Could you check a few things on this model? Use its own coordinates, in mm. Face numbers are marked on the shaded views. A direction names the side the tool comes from. Give positions to 0.01 mm unless a question says otherwise; leave off trailing zeros. Write each loop counter-clockwise with the first axis right and the second up, starting at its lowest first coordinate (ties: lowest second). Pieces come first, ordered by that corner, then holes. Notation, with made-up numbers: M -39.5,75.25 L 7.5,75.25 A11 cw 7.5,84.25 Z; hole C 25,-26.75 d1. An arc over 180 degrees is marked long. Use one line per item in the form item = value.
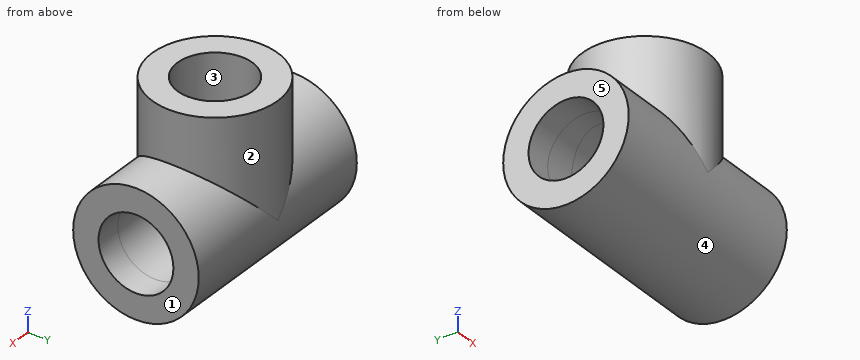
from build123d import *

# Parameters (mm, degrees)
F0_R          = 19
F0_R_2        = 11.335
F1_DEPTH      = 33
F1_DEPTH_BACK = 33
F2_R          = 19
F2_R_2        = 11.335
F3_DEPTH      = 34.5
F4_DEPTH      = 25
F4_DEPTH_BACK = 25


with BuildPart() as f1:
    # F0 (on Right) → F1 (new body, two sides)
    with BuildSketch(Plane.YZ) as f1_sk:
        Circle(F0_R)
        Circle(F0_R_2, mode=Mode.SUBTRACT)
    extrude(amount=F1_DEPTH)
    extrude(f1_sk.sketch, amount=-F1_DEPTH_BACK)

    # F2 (on Top) → F3 (join)
    with BuildSketch(Plane.XY):
        Circle(F2_R)
        Circle(F2_R_2, mode=Mode.SUBTRACT)
    extrude(amount=F3_DEPTH)

    # F0 (on Right) → F4 (cut, two sides)
    with BuildSketch(Plane.YZ) as f4_sk:
        Circle(F0_R_2)
    extrude(amount=-F4_DEPTH, mode=Mode.SUBTRACT)
    extrude(f4_sk.sketch, amount=F4_DEPTH_BACK, mode=Mode.SUBTRACT)


solid = f1.part
1) If I drill on L1, parallel to Z at x = 9.5, y = 0 (3 decimals), over which ranges is the centre line in solid material (lowest first)?
Checked values:
L1 = -19 to -11.335, 11.335 to 19
2) Thinking about a two-plate mould opening in Y: for the marked faces 1, 2 and 3, which applies, released by +Y, released by -Y, zero draft, split by the parting line, or undercut?
Checked values:
face_1 = zero draft
face_2 = split by the parting line
face_3 = undercut
3) For the marked faces 4 and 5, which set-ups out of +Z, -Z, +X, -X, +Y, -Y let a thin tool reach every point of the face, with its end or its side?
Checked values:
face_4 = none
face_5 = +Z, -Z, -X, +Y, -Y
4) I want a section at D-D, the plane x = -3.5. Please give me the cut outline in (y, z) (3 decimals), plus the area to 3 significant figures.
Checked values:
outline = M -18.675,3.5 A19 ccw long 18.675,3.5 L 18.675,34.5 L 10.781,34.5 L 10.781,15.645 A19 ccw -10.781,15.645 L -10.781,34.5 L -18.675,34.5 Z; hole C 0,0 d22.67
area = 1,100 mm2
5) I want a section at A-A, the plane y = 0. Please give me the cut outline in (x, z) (3 decimals), plus the area to 3 significant figures.
Checked values:
outline = M -33,-19 L 33,-19 L 33,-11.335 L -33,-11.335 Z; M -33,11.335 L 33,11.335 L 33,19 L 19,19 L 19,34.5 L 11.335,34.5 L 11.335,19 L -11.335,19 L -11.335,34.5 L -19,34.5 L -19,19 L -33,19 Z
area = 1,250 mm2
6) I want a section at C-C, the plane z = 26. Please give me the cut outline in (x, y) (3 decimals).
Checked values:
outline = C 0,0 d38; hole C 0,0 d22.67
7) I want a section at B-B, the plane z = 10.5. Please give me the cut outline in (x, y).
Checked values:
outline = M -33,-15.84 L -10.5,-15.84 A19 ccw 10.5,-15.84 L 33,-15.84 L 33,-4.27 L -33,-4.27 Z; M -33,4.27 L 33,4.27 L 33,15.84 L 10.5,15.84 A19 ccw -10.5,15.84 L -33,15.84 Z
8) For pin 1 Ø8 at (y, z) = (8, 28.5) entering from +X; pin 2 Ø1.5 at (y, z) = (14, 25.5) entering from +X; pin 3 Ø6 at (y, z) = (8.5, -4) entering from +X; pin 4 Ø8 at (x, z) = (-12, -13.5) entering from -Y, each with a flat end and sliding along its axis, tell me the tip position at first contact or that it passes through.
Checked values:
pin_1 = 18.57
pin_2 = 13.62
pin_3 = 33
pin_4 = -16.45
